For this review, use the dimensioned drawing (mm, ordinates from the lowest corner) and the shaded views. A direction names the side the tool comes from. Coordinates: 2 decimals unless noted, no trailing zeros. Order: outer loops, then holes, each group sorted by start corner. A loop starts at its lowest first (then second) coordinate and runs counter-clockwise, first axis right, second up. Notation, with made-up numbers: (19, -0.5) -> (62, -0.5) arc R16 ccw to (62, 26.5) -> close; hole circle Ø8 at (76.25, 45.25). An arc over 180 degrees is marked (long way). Return JSON: item names as keys, results as strings. Group by question number.
Item 1: Machinability: for the marked faces 1, 2 and 3, which of the approach directions +Z, -Z, +X, -X, +Y, -Y give a long, thin tool a straight path to every point of the face, cutting with its end or side? Answer none if there is none.
Item 2: Take a section at C-C (x = 18.5). Write out the cut boundary in (y, z).
Item 3: Insertion check: pin 1 (8 mm diameter, centred on y = 17, z = 16, fed in from -X); pin 2 (2.5 mm diameter, centred on x = 26.99, y = 3.62, fed in from +Z); pin 3 (2 mm diameter, centred on x = 8.5, y = 3, fed in from +Z). Each pin has a flat end and moves straight along its axis. Give the tip position at first contact, or say it passes through.
Item 4: Take a section at D-D (x = 3.25). Write out the cut boundary in (y, z).
Item 5: Take a section at A-A (y = 15). Write out the cut boundary in (x, z), then the cut area to 3 significant figures.
Item 6: For line 1 along X through (y, z) = (17.5, 18); line 2 along Y through (x, z) = (18.25, 22); line 3 along Y through (x, z) = (18.25, 23.5), list the stretches that pass through material, from the lowest coordinate up.
Item 7: Take a section at B-B (z = 22). Write out the cut boundary in (x, y), then the cut area to 3 significant figures.
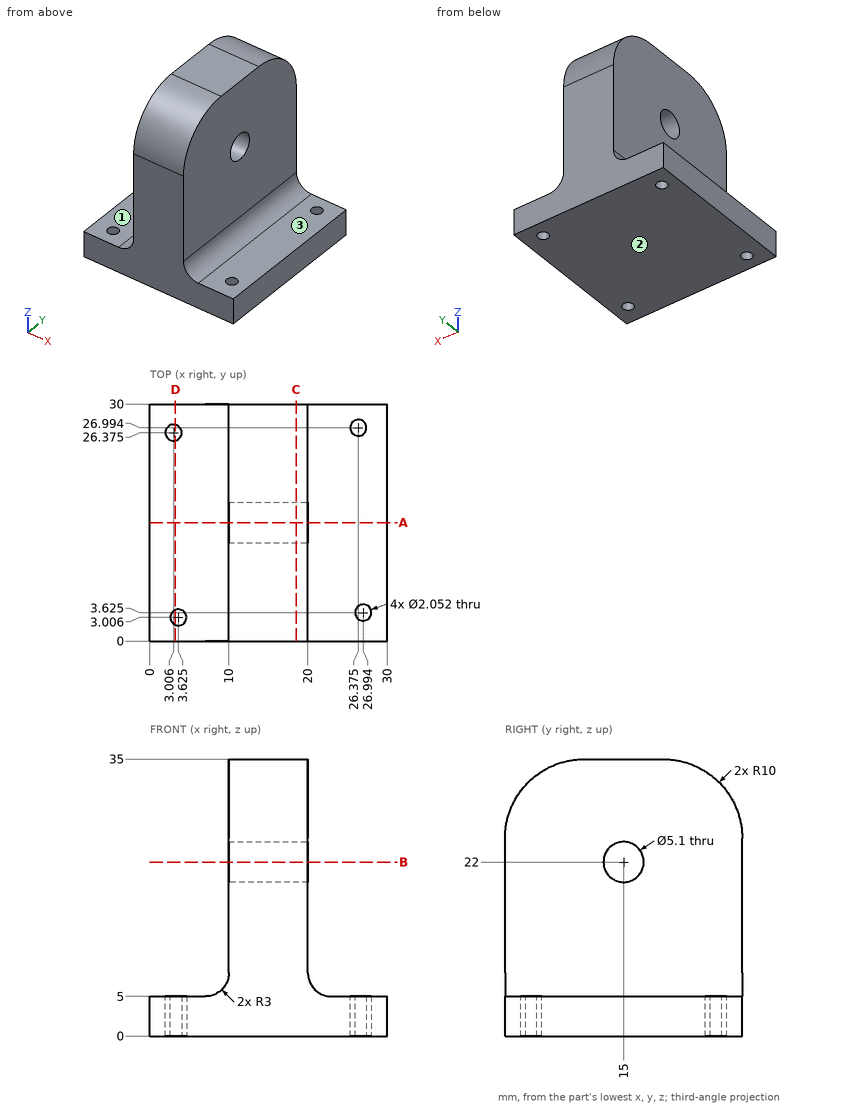
Findings below:
{
 "1": {"face 1": "+Z, -X, +Y, -Y", "face 2": "-Z, +X, -X, +Y, -Y", "face 3": "+Z, +X, +Y, -Y"},
 "2": {"outline": "(0, 0) -> (30, 0) -> (30, 25) arc R10 ccw to (20, 35) -> (10, 35) arc R10 ccw to (0, 25) -> close; hole circle Ø5.1 at (15, 22)"},
 "3": {"pin 1": "stops at x = 10", "pin 2": "stops at z = 5", "pin 3": "stops at z = 6.34"},
 "4": {"outline": "(0, 0) -> (2.05, 0) -> (2.05, 5) -> (0, 5) -> close; (3.96, 0) -> (25.38, 0) -> (25.38, 5) -> (3.96, 5) -> close; (27.37, 0) -> (30, 0) -> (30, 5) -> (27.37, 5) -> close"},
 "5": {"outline": "(0, 0) -> (30, 0) -> (30, 5) -> (23, 5) arc R3 cw to (20, 8) -> (20, 19.45) -> (10, 19.45) -> (10, 8) arc R3 cw to (7, 5) -> (0, 5) -> close; (10, 24.55) -> (20, 24.55) -> (20, 35) -> (10, 35) -> close", "area": "403 mm2"},
 "6": {"line 1": "x = 10 to 20", "line 2": "y = 0 to 12.45, 17.55 to 30", "line 3": "y = 0 to 12.94, 17.06 to 30"},
 "7": {"outline": "(10, 0) -> (20, 0) -> (20, 12.45) -> (10, 12.45) -> close; (10, 17.55) -> (20, 17.55) -> (20, 30) -> (10, 30) -> close", "area": "249 mm2"}
}
